Read the model definition and answer for the solid it produces. Units are mm, in the model's axes. Face numbers are marked on the shaded views. Round coordinates to 2 decimals unless told otherwise and drop trailing zeros. Write each loop counter-clockwise with the first axis right and the second up, starting at its lowest first coordinate (ties: lowest second). Pieces come first, ordered by that corner, then holes. Notation, with made-up numbers: (17.5, -39.5) -> (64.5, -39.5) arc R34 cw to (64.5, -2.5) -> close; hole circle Ø4 at (-1, 14). An arc over 180 degrees is marked (long way). Return JSON: item names as keys, results as strings. Group by question number.
(1) Straight lines are drawn through the part: line 1 (Z direction, x = 0, y = -0.25); line 2 (Z direction, x = 0, y = -1.35); line 3 (Z direction, x = 2.75, y = -3.15). For each, find the intervals that lie inside material, in ascending order.
(2) A cutting plane is placed at D-D on y = -3.7. Give the vertices of the cut face in (x, z).
(3) A cutting plane is placed at C-C on x = -1.75. Give the vertices of the cut face in (y, z).
(4) The mould has two halves that part along Z. Classify the marked faces 1, 2 and 3: released by +Z, released by -Z, zero draft, split by the parting line, or undercut.
(5) A cutting plane is placed at A-A on z = 0. Give the vertices of the cut face in (x, y), then the cut area to 3 significant figures.
(6) A cutting plane is placed at B-B on x = 0. Give the vertices of the cut face in (y, z), then the cut area to 3 significant figures.
(7) Given pin 1 (6.5 mm diameter, centred on x = 1.5, z = -9.5, fed in from -Y); pin 2 (0.5 mm diameter, centred on y = -0.5, z = 8, fed in from -X); pin 3 (0.5 mm diameter, centred on y = -0.5, z = -7.5, fed in from +X), each flat-ended and moving along its own axis, determine where each tip first touches the part or whether it passes through.
```python
from build123d import *

# Parameters (mm, degrees)
F0_W        = 4.5
F0_H        = 5
F3_DEPTH    = 1
F4_W        = 10
F4_H        = 4
F5_DEPTH    = 1
F6_T1_DEPTH = 1
F7_R        = 3
F8_DEPTH    = 4.501


# Not quite as in the source:
# - a fillet or chamfer that OpenCascade refuses, or shapes differently, is made with other operations: its cross-section is extruded or revolved along the edge and cut away or added


with BuildPart() as f1:
    # F0 (on Right) → F1 (revolve)
    with BuildSketch(Plane.YZ):
        with Locations((-2.25, 2.5)):
            Rectangle(F0_W, F0_H)
    revolve(axis=Axis((0, -2.25, 0), (0, -1, 0)))

    # F2 (on face) → F3 (join)
    with BuildSketch(Plane(origin=(0, 0, 0), x_dir=(-1, 0, 0), z_dir=(0, 1, 0))):
        with BuildLine():
            ThreePointArc((-2.5, -10), (0, -12.5), (2.5, -10))
            Line((2.5, -10), (1.05, -10))
            ThreePointArc((1.05, -10), (0, -11.05), (-1.05, -10))
            Line((-1.05, -10), (-2.5, -10))
        make_face()
        with BuildLine():
            Line((1.05, -10), (2.5, -10))
            Line((2.5, -10), (2.5, 10))
            Line((2.5, 10), (1.05, 10))
            ThreePointArc((1.05, 10), (0, 8.95), (-1.05, 10))
            Line((-1.05, 10), (-2.5, 10))
            Line((-2.5, 10), (-2.5, -10))
            Line((-2.5, -10), (-1.05, -10))
            ThreePointArc((-1.05, -10), (0, -8.95), (1.05, -10))
        make_face()
        with BuildLine():
            Line((1.05, 10), (2.5, 10))
            ThreePointArc((2.5, 10), (0, 12.5), (-2.5, 10))
            Line((-2.5, 10), (-1.05, 10))
            ThreePointArc((-1.05, 10), (0, 11.05), (1.05, 10))
        make_face()
    extrude(amount=-F3_DEPTH)

    # F4 (on face) → F5 (join)
    with BuildSketch(Plane(origin=(0, 0, 0), x_dir=(-1, 0, 0), z_dir=(0, 1, 0))):
        Rectangle(F4_W, F4_H)
        with BuildLine():
            Line((5, 2), (5, -2))
            ThreePointArc((5, -2), (7, 0), (5, 2))
        make_face()
        with BuildLine():
            ThreePointArc((-5, 2), (-7, 0), (-5, -2))
            Line((-5, -2), (-5, 2))
        make_face()
    extrude(amount=-F5_DEPTH)

    # F6: fillet of radius 1 on 8 edges, made by hand

    # F6_s2 → F6_t1 (join)
    with BuildSketch(Plane.XZ):
        with BuildLine():
            ThreePointArc((-2.5, 4.8733971724), (-2.610243479, 4.4169617078), (-2.9166666667, 4.0611643103))
            ThreePointArc((-2.9166666667, 4.0611643103), (-2.7116700904, 4.2008148401), (-2.5, 4.3301270189))
            Line((-2.5, 4.3301270189), (-2.5, 4.8733971724))
        make_face()
        with BuildLine():
            ThreePointArc((-2.9166666667, -4.0611643103), (-2.610243479, -4.4169617078), (-2.5, -4.8733971724))
            Line((-2.5, -4.8733971724), (-2.5, -4.3301270189))
            ThreePointArc((-2.5, -4.3301270189), (-2.7116700904, -4.2008148401), (-2.9166666667, -4.0611643103))
        make_face()
        with BuildLine():
            ThreePointArc((4.3333333333, 2.4944382578), (4.6708497378, 2.144797772), (5.1333333333, 1.9955506063))
            Line((5.1333333333, 1.9955506063), (5.1266666667, 1.895773076))
            ThreePointArc((5.1266666667, 1.895773076), (5, 1.9), (4.582575695, 1.9))
            Line((4.582575695, 1.9), (4.4909241811, 1.96))
            ThreePointArc((4.4909241811, 1.96), (4.3755080286, 2.2056585166), (4.2466666667, 2.4445494927))
            Line((4.2466666667, 2.4445494927), (4.3333333333, 2.4944382578))
        make_face()
        with BuildLine():
            ThreePointArc((-4.3333333333, 2.4944382578), (-4.6708497378, 2.144797772), (-5.1333333333, 1.9955506063))
            Line((-5.1333333333, 1.9955506063), (-5.1266666667, 1.895773076))
            ThreePointArc((-5.1266666667, 1.895773076), (-5, 1.9), (-4.582575695, 1.9))
            Line((-4.582575695, 1.9), (-4.4909241811, 1.96))
            ThreePointArc((-4.4909241811, 1.96), (-4.3755080286, 2.2056585166), (-4.2466666667, 2.4445494927))
            Line((-4.2466666667, 2.4445494927), (-4.3333333333, 2.4944382578))
        make_face()
        with BuildLine():
            ThreePointArc((4.3333333333, -2.4944382578), (4.6708497378, -2.144797772), (5.1333333333, -1.9955506063))
            Line((5.1333333333, -1.9955506063), (5.1266666667, -1.895773076))
            ThreePointArc((5.1266666667, -1.895773076), (5, -1.9), (4.582575695, -1.9))
            Line((4.582575695, -1.9), (4.4909241811, -1.96))
            ThreePointArc((4.4909241811, -1.96), (4.3755080286, -2.2056585166), (4.2466666667, -2.4445494927))
            Line((4.2466666667, -2.4445494927), (4.3333333333, -2.4944382578))
        make_face()
        with BuildLine():
            ThreePointArc((-4.3333333333, -2.4944382578), (-4.6708497378, -2.144797772), (-5.1333333333, -1.9955506063))
            Line((-5.1333333333, -1.9955506063), (-5.1266666667, -1.895773076))
            ThreePointArc((-5.1266666667, -1.895773076), (-5, -1.9), (-4.582575695, -1.9))
            Line((-4.582575695, -1.9), (-4.4909241811, -1.96))
            ThreePointArc((-4.4909241811, -1.96), (-4.3755080286, -2.2056585166), (-4.2466666667, -2.4445494927))
            Line((-4.2466666667, -2.4445494927), (-4.3333333333, -2.4944382578))
        make_face()
        with BuildLine():
            ThreePointArc((2.9166666667, 4.0611643103), (2.610243479, 4.4169617078), (2.5, 4.8733971724))
            Line((2.5, 4.8733971724), (2.5, 4.3301270189))
            ThreePointArc((2.5, 4.3301270189), (2.7116700904, 4.2008148401), (2.9166666667, 4.0611643103))
        make_face()
        with BuildLine():
            ThreePointArc((2.9166666667, -4.0611643103), (2.610243479, -4.4169617078), (2.5, -4.8733971724))
            Line((2.5, -4.8733971724), (2.5, -4.3301270189))
            ThreePointArc((2.5, -4.3301270189), (2.7116700904, -4.2008148401), (2.9166666667, -4.0611643103))
        make_face()
    extrude(amount=F6_T1_DEPTH)

    # F7 (on face) → F8 (cut, through all)
    with BuildSketch(Plane(origin=(0, 0, 0), x_dir=(-1, 0, 0), z_dir=(0, 1, 0))):
        Circle(F7_R)
    extrude(amount=-F8_DEPTH, mode=Mode.SUBTRACT)


solid = f1.part
```
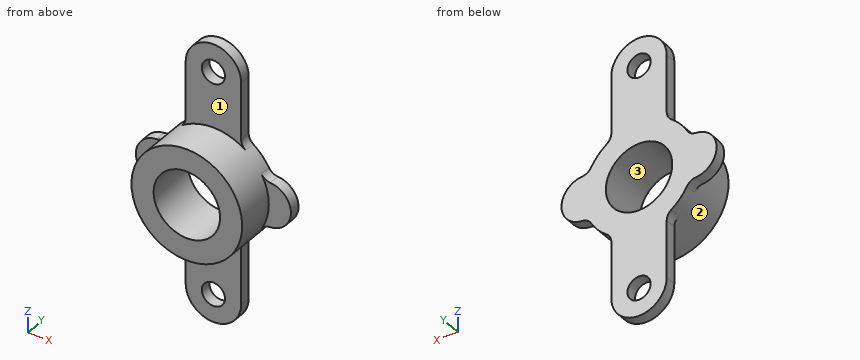
Checks:
{
 "1": {"line 1": "z = -12.5 to -11.05, -8.95 to -3, 3 to 8.95, 11.05 to 12.5", "line 2": "z = -5 to -3, 3 to 5", "line 3": "z = -4.18 to -1.2, 1.2 to 4.18"},
 "2": {"outline": "circle Ø10 at (0, 0); hole circle Ø6 at (0, 0)"},
 "3": {"outline": "(-4.5, -4.68) -> (-1, -4.68) -> (-1, -11.79) -> (0, -11.79) -> (0, -2.44) -> (-4.5, -2.44) -> close; (-4.5, 2.44) -> (0, 2.44) -> (0, 11.79) -> (-1, 11.79) -> (-1, 4.68) -> (-4.5, 4.68) -> close"},
 "4": {"face 1": "zero draft", "face 2": "split by the parting line", "face 3": "undercut"},
 "5": {"outline": "(-7, -1) -> (-5, -1) -> (-5, -4.5) -> (-3, -4.5) -> (-3, 0) -> (-7, 0) -> close; (3, -4.5) -> (5, -4.5) -> (5, -1) -> (7, -1) -> (7, 0) -> (3, 0) -> close", "area": "22.0 mm^2"},
 "6": {"outline": "(-4.5, -5) -> (-1, -5) -> (-1, -8.95) -> (0, -8.95) -> (0, -3) -> (-4.5, -3) -> close; (-4.5, 3) -> (0, 3) -> (0, 8.95) -> (-1, 8.95) -> (-1, 5) -> (-4.5, 5) -> close; (-1, -12.5) -> (0, -12.5) -> (0, -11.05) -> (-1, -11.05) -> close; (-1, 11.05) -> (0, 11.05) -> (0, 12.5) -> (-1, 12.5) -> close", "area": "28.8 mm^2"},
 "7": {"pin 1": "stops at y = -1", "pin 2": "stops at x = -2.5", "pin 3": "stops at x = 2.5"}
}
